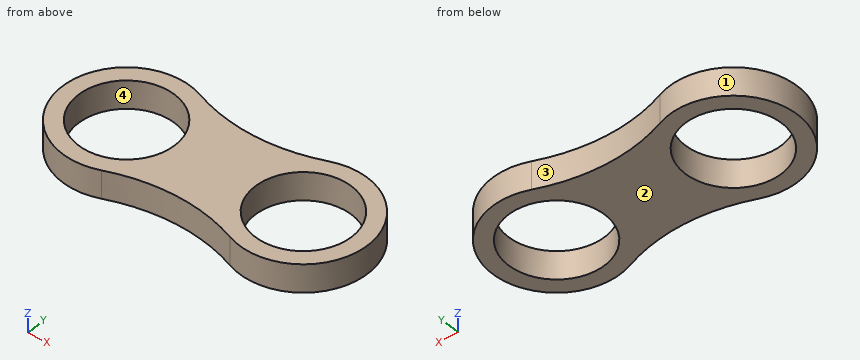
```python
from build123d import *

# Parameters (mm, degrees)
F0_R     = 11.25
F1_DEPTH = 6.55


with BuildPart() as f1:
    # F0 (on Top) → F1 (new body)
    with BuildSketch(Plane.XY):
        with BuildLine():
            ThreePointArc((-35.367126, -13.902184), (-20.5, -11.004665), (-5.632874, -13.902184))
            ThreePointArc((-5.632874, -13.902184), (15, 0), (-5.632874, 13.902184))
            ThreePointArc((-5.632874, 13.902184), (-20.5, 11.004665), (-35.367126, 13.902184))
            ThreePointArc((-35.367126, 13.902184), (-56, 0), (-35.367126, -13.902184))
        make_face()
        with Locations((-41, 0)):
            Circle(F0_R, mode=Mode.SUBTRACT)
        Circle(F0_R, mode=Mode.SUBTRACT)
    extrude(amount=F1_DEPTH)


solid = f1.part
```
Design review of the part built by this model. Coordinates are the model's own, in mm. Face numbers are marked on the shaded views. Round coordinates to 2 decimals unless told otherwise and drop trailing zeros. Write each loop counter-clockwise with the first axis right and the second up, starting at its lowest first coordinate (ties: lowest second). Pieces come first, ordered by that corner, then holes. Notation, with made-up numbers: (55.5, 19) -> (82.5, 19) arc R24 cw to (82.5, 37) -> close; hole circle Ø3 at (61, -39). An arc over 180 degrees is marked (long way). Answer in a Markdown table with one row per item.
Q1. Clearance check with flat-ended pins moving along their axes: pin 1 Ø2 at (x, z) = (4.5, 2) entering from -Y; pin 2 Ø5 at (x, y) = (6, 3) entering from +Z. State where each tip first meets the part, or that it passes through.
The answers:
| item | result |
|---|---|
| pin 1 | y = -14.59 |
| pin 2 | through |
Q2. To check wall thickness, follow L1, parallel to X at y = 0.25, z = 2.25; L2, parallel to Y at x = -41, z = 2.5; L3, parallel to X at y = 10.25, z = 1.5. State the ranges of each line that lie inside material, in increasing order. Write a range as [from, to].
The answers:
| item | result |
|---|---|
| L1 | [-56, -52.25], [-29.75, -11.25], [11.25, 15] |
| L2 | [-15, -11.25], [11.25, 15] |
| L3 | [-51.95, -45.64], [-36.36, -4.64], [4.64, 10.95] |
Q3. Take a section at D-D, the plane y = 10. State the section outline as (x, z) points, then the cut area to 3 significant figures.
The answers:
| item | result |
|---|---|
| outline | (-52.18, 0) -> (-46.15, 0) -> (-46.15, 6.55) -> (-52.18, 6.55) -> close; (-35.85, 0) -> (-5.15, 0) -> (-5.15, 6.55) -> (-35.85, 6.55) -> close; (5.15, 0) -> (11.18, 0) -> (11.18, 6.55) -> (5.15, 6.55) -> close |
| area | 280 mm² |
Q4. Take a section at B-B, the plane x = 0. State the section outline as (y, z) points.
The answers:
| item | result |
|---|---|
| outline | (-15, 0) -> (-11.25, 0) -> (-11.25, 6.55) -> (-15, 6.55) -> close; (11.25, 0) -> (15, 0) -> (15, 6.55) -> (11.25, 6.55) -> close |
Q5. Take a section at C-C, the plane z = 3.25. State the section outline as (x, y) points, then the cut area to 3 significant figures.
The answers:
| item | result |
|---|---|
| outline | (-35.37, -13.9) arc R39.59 cw to (-5.63, -13.9) arc R15 ccw (long way) to (-5.63, 13.9) arc R39.59 cw to (-35.37, 13.9) arc R15 ccw (long way) to start; hole circle Ø22.5 at (-41, 0); hole circle Ø22.5 at (0, 0) |
| area | 952 mm² |
Q6. Draft analysis for pull direction Y (two halves, no side actions). For the marked faces 1, 2, 3 and 4, state which applies: +Y half, -Y half, draft (parallel to the pull), parting line (faces both ways), or undercut.
The answers:
| item | result |
|---|---|
| face 1 | parting line |
| face 2 | draft |
| face 3 | +Y half |
| face 4 | undercut |
Q7. Take a section at A-A, the plane y = 0. State the section outline as (x, z) points, then the cut area to 3 significant figures.
The answers:
| item | result |
|---|---|
| outline | (-56, 0) -> (-52.25, 0) -> (-52.25, 6.55) -> (-56, 6.55) -> close; (-29.75, 0) -> (-11.25, 0) -> (-11.25, 6.55) -> (-29.75, 6.55) -> close; (11.25, 0) -> (15, 0) -> (15, 6.55) -> (11.25, 6.55) -> close |
| area | 170 mm² |
